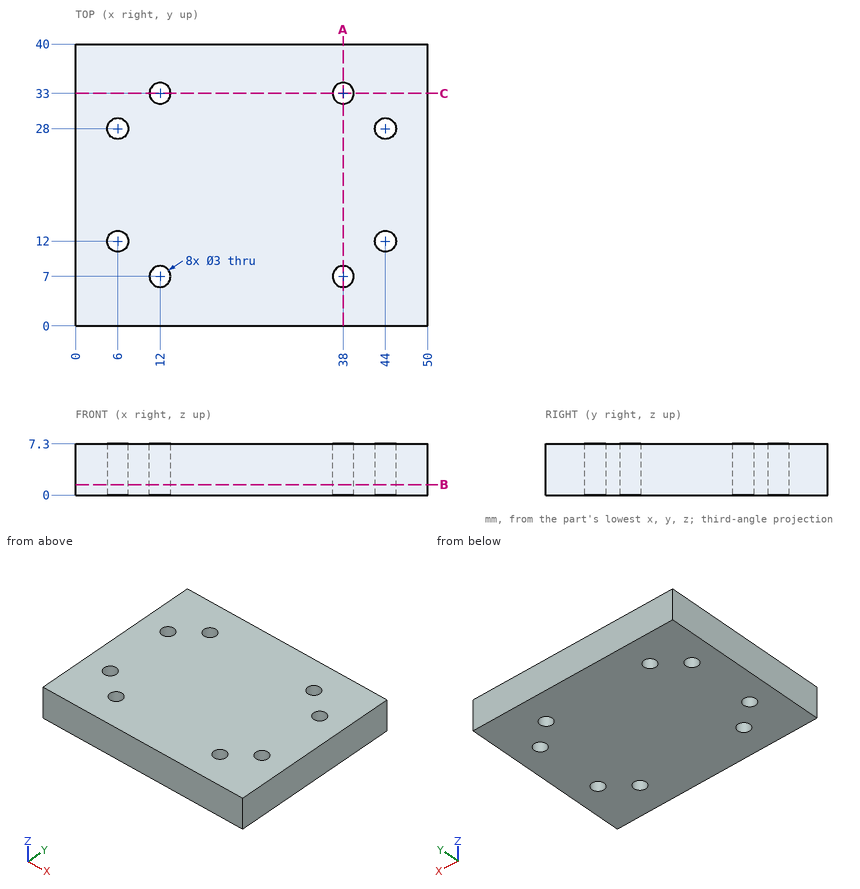
The figure shows three views and two pictorial views of one solid part (mm, origin at its lowest corner). Answer the questions. Give positions to 0.01 mm unless a question says otherwise; leave off trailing zeros. Loops run counter-clockwise (first coordinate to the right, second up) from the corner with the lowest first, then second, coordinate; pieces in that order, holes last. Notation, with made-up numbers: (38, 74.5) -> (71, 74.5) arc R18 ccw to (71, 88.5) -> close; hole circle Ø9 at (-30.75, 55). An arc over 180 degrees is marked (long way). Use CSV: the item, a comma, the result in double quotes.
1. Straight lines are drawn through the part: line 1 (Y direction, x = 12, z = 2.75); line 2 (X direction, y = 12, z = 3.25); line 3 (Y direction, x = 44, z = 1.75). For each, find the intervals that lie inside material, in ascending order.
Found:
line 1,"0 to 5.5, 8.5 to 31.5, 34.5 to 40"
line 2,"0 to 4.5, 7.5 to 42.5, 45.5 to 50"
line 3,"0 to 10.5, 13.5 to 26.5, 29.5 to 40"
2. A flat-ended cylindrical pin translates along its axis: pin 1 Ø1.8 at (x, y) = (6, 28) entering from +Z. Find the tip coordinate at first contact, or state that the pin passes through.
Found:
pin 1,"through"
3. The part is cut by section C-C (y = 33). Write down the section's boundary in (x, z).
Found:
outline,"(0, 0) -> (10.5, 0) -> (10.5, 7.3) -> (0, 7.3) -> close; (13.5, 0) -> (36.5, 0) -> (36.5, 7.3) -> (13.5, 7.3) -> close; (39.5, 0) -> (50, 0) -> (50, 7.3) -> (39.5, 7.3) -> close"
4. The part is cut by section B-B (z = 1.5). State how many separate pieces and enclosed holes the cut face has, then the cut area to 3 significant figures.
Found:
separate pieces,"1"
enclosed holes,"8"
area,"1,940 mm^2"
5. The part is cut by section A-A (x = 38). Write down the section's boundary in (y, z), then the cut area to 3 significant figures.
Found:
outline,"(0, 0) -> (5.5, 0) -> (5.5, 7.3) -> (0, 7.3) -> close; (8.5, 0) -> (31.5, 0) -> (31.5, 7.3) -> (8.5, 7.3) -> close; (34.5, 0) -> (40, 0) -> (40, 7.3) -> (34.5, 7.3) -> close"
area,"248 mm^2"
